Here's how the part is built. I have some questions about the finished solid (model axes, mm). A direction names the side the tool comes from. Give positions to 0.01 mm unless a question says otherwise; leave off trailing zeros. Loops run counter-clockwise (first coordinate to the right, second up) from the corner with the lowest first, then second, coordinate; pieces in that order, holes last. Notation, with made-up numbers: (35.25, 22) - (59.25, 22) arc R17 ccw to (59.25, 51) - close; hole circle Ø9 at (38, -8). An arc over 180 degrees is marked (long way). Return JSON: item names as keys, results as strings. Group by question number.
(1) For P1, Ø5, axis at y = -2.5, z = -18.5, coming from the -X side; P2, Ø16, axis at y = 2, z = -5.5, coming from the -X side; P3, Ø10, axis at y = 24, z = 14, coming from the +X side; P4, Ø9.5, axis at y = 0, z = 0, coming from the -X side, each with a flat end and sliding along its axis, tell me the tip position at first contact or that it passes through.
(2) On a 3-axis mill with a long thin cutter (end or side, diameter ignored), from which of +Z, -Z, +X, -X, +Y, -Y can I reach the whole of each face in a straight line? I mean faces 4 (the flat face through (85, 15, -3)), 5 (the cylindrical face through (0.74, -7.509, 23.846)), 6 (the flat face through (16.5, 9, -9)), 7 (the cylindrical face through (22.862, 30.736, -4.036)). Say none if no direction works.
(3) I need wall thicknesses on probe 1 along Z at (x, y) = (19, 0); probe 2 along Y at (x, z) = (26.75, 0); probe 3 along X at (y, z) = (11.5, -15). Which ranges of each line are inside material? Lowest first, please. Write a range as [from, to].
(4) If we mould it in two halves opening along X, with no side actions, what happens to faces 1 (the flat face through (1.5, 16.3, 0.3)), 2 (the flat face through (22, 11, -12)), 3 (the flat face through (68, -15.3, -13.4))? For each: released by +X, released by -X, zero draft, split by the parting line, or undercut.
(5) If we section it at B-B (x = 11.5): Please give me the cut outline in (y, z).
(6) If we section it at A-A (x = 73.5): Please give me the cut outline in (y, z), then the cut area to 3 significant figures.
```python
from build123d import *

# Parameters (mm, degrees)
F4_R = 5.99999
F5_R = 5
F6_R = 5


# Not quite as in the source:
# - a fillet or chamfer is up to 0.001 mm smaller than in the source, because OpenCascade refuses the exact size


with BuildPart() as f1:
    # F0 (on Front) → F1 (revolve)
    with BuildSketch(Plane.XZ):
        with BuildLine():
            Line((0, 31), (0, 0))
            Line((0, 0), (88, 0))
            Line((88, 0), (88, 15))
            Line((88, 15), (85, 15))
            Line((85, 15), (85, 20))
            Line((85, 20), (68, 20))
            Line((68, 20), (68, 31))
            Line((68, 31), (56, 31))
            ThreePointArc((56, 31), (50, 25), (44, 31))
            Line((44, 31), (0, 31))
        make_face()
    revolve(axis=Axis((44, 0, 0), (-1, 0, 0)))

    # F2 (on Front) → F3 (revolve, cut)
    with BuildSketch(Plane.XZ):
        Polygon((0, 25), (0, 0), (88, 0), (88, 6), (30, 6), (30, 16), (22, 16), (22, 20.5), (16.5, 20.5), (16.5, 12.5), (13.5, 12.5), (13.5, 16), (1.5, 16), (1.5, 25), align=None)
    revolve(axis=Axis((44.884205035, 0, 0), (1, 0, 0)), mode=Mode.SUBTRACT)

    # F4 (radius 6 in the source; OpenCascade refuses exactly that, so slightly less here)
    f4_edges = [f1.edges().sort_by_distance(p)[0] for p in [
        (0, 0, -31),
    ]]
    fillet(f4_edges, radius=F4_R)

    # F5
    f5_edges = [f1.edges().sort_by_distance(p)[0] for p in [
        (44, 0, -31),
        (56, 0, -31),
    ]]
    fillet(f5_edges, radius=F5_R)

    # F6
    f6_edges = [f1.edges().sort_by_distance(p)[0] for p in [
        (68, 0, -31),
    ]]
    fillet(f6_edges, radius=F6_R)


solid = f1.part
```
Values:
{
 "1": {"P1": "x = 1.5", "P2": "x = 13.5", "P3": "x = 68", "P4": "through"},
 "2": {"face 4": "+X", "face 5": "-X", "face 6": "none", "face 7": "+X, -X"},
 "3": {"probe 1": "[-31, -20.5], [20.5, 31]", "probe 2": "[-31, -16], [16, 31]", "probe 3": "[1.5, 16.5], [22, 85]"},
 "4": {"face 1": "released by -X", "face 2": "undercut", "face 3": "released by +X"},
 "5": {"outline": "circle Ø62 at (0, 0); hole circle Ø32 at (0, 0)"},
 "6": {"outline": "circle Ø40 at (0, 0); hole circle Ø12 at (0, 0)", "area": "1,140 mm2"}
}
